The listing builds one solid part. Answer for the finished solid, in the listing's coordinates (mm). A direction names the side the tool comes from. Coordinates: 2 decimals unless noted, no trailing zeros. Order: outer loops, then holes, each group sorted by start corner. A loop starts at its lowest first (then second) coordinate and runs counter-clockwise, first axis right, second up. Notation, with made-up numbers: (34.5, 11) -> (70.5, 11) arc R18 ccw to (70.5, 39) -> close; hole circle Ø1 at (22.25, -36). An arc over 180 degrees is marked (long way). Put each result on its own line as item: value. Start each with the question number.
Autodesk Inventor part; units mm, degrees
ref_plane "YZ Plane" through (0, 0, 0) normal (1, 0, 0) x (0, 1, 0)
ref_plane "XZ Plane" through (0, 0, 0) normal (0, 1, 0) x (-1, 0, 0)
ref_plane "XY Plane" through (0, 0, 0) normal (0, 0, 1) x (1, 0, 0)
sketch "Boceto1" plane through (0, 0, 0) normal (0, 1, 0) x (-1, 0, 0)
  line L0 (20.5, -20.5) -> (-20.5, -20.5)
  line L1 (-20.5, -20.5) -> (-20.5, 20.5)
  line L2 (-20.5, 20.5) -> (20.5, 20.5)
  line L3 (20.5, 20.5) -> (20.5, -20.5)
  point P0 (0, 0)
  point P1 (0, -20.5)
  point P2 (-20.5, 0)
  dimension "d0" = 41
  dimension "d1" = 41
extrude "Extrusión1" add sketch "Boceto1" along normal blind 94
sketch "Boceto2" plane through (0, 94, 0) normal (0, 1, 0) x (1, 0, 0)
  line L0 (20.5, 20.5) -> (-20.5, 20.5)
  line L1 (-20.5, 20.5) -> (59.5, 20.5)
  line L2 (59.5, 20.5) -> (59.5, 6.5)
  line L3 (-20.5, -20.5) -> (20.5, -20.5)
  line L4 (59.5, 6.5) -> (20.5, -20.5)
  line L5 (20.5, -20.5) -> (20.5, 20.5)
  line L6 (50.8333, 0.5) -> (20.5, 0.5)
  line L7 (22.5, 18.5) -> (57.5, 18.5)
  line L8 (57.5, 18.5) -> (57.5, 7.5479)
  line L9 (57.5, 7.5479) -> (50.2086, 2.5)
  line L10 (22.5, 18.5) -> (22.5, 2.5)
  line L11 (22.5, 2.5) -> (50.2086, 2.5)
  line L12 (22.5, 0.5) -> (22.5, -16.6829)
  line L13 (22.5, -16.6829) -> (47.3197, 0.5)
  point P0 (0, 0)
  point P1 (36.3543, 2.5)
  dimension "d4" = 80
  dimension "d5" = 14
  dimension "d9" = 2
  dimension "d10" = 2
  dimension "d11" = 2
  dimension "d12" = 2
  dimension "d13" = 2
  dimension "d20" = 5.0479
extrude "Extrusión2" add sketch "Boceto2" along normal blind 8 contours L1 L2 L4 L6 L5 | L6 L12 L13 L4 L5
sketch "Boceto3" plane through (0, 94, 0) normal (0, 1, 0) x (1, 0, 0)
  line L0 (-20.5, 20.5) -> (-20.5, -20.5)
  line L1 (20.5, -20.5) -> (59.5, 6.5)
  line L2 (-20.5, 20.5) -> (20.5, 20.5)
  line L3 (20.5, 20.5) -> (20.5, -20.5)
  line L4 (20.5, -20.5) -> (-20.5, -20.5)
  line L5 (-20.5, -20.5) -> (-20.5, 20.5)
  point P0 (0, 0)
extrude "Extrusión3" add sketch "Boceto3" along normal blind 8
sketch "Boceto4" plane through (0, 102, 0) normal (0, 1, 0) x (1, 0, 0)
  point P0 (0, 0)
sketch "Boceto6" plane through (0, 102, 0) normal (0, 1, 0) x (1, 0, 0)
  line L0 (-20.5, 20.5) -> (-20.5, -20.5)
  line L1 (59.5, 6.5) -> (59.5, 20.5)
  line L2 (-20.5, 20.5) -> (59.5, 20.5)
  line L3 (59.5, 20.5) -> (59.5, 6.5)
  line L4 (20.5, -20.5) -> (59.5, 6.5)
  line L5 (59.5, 6.5) -> (20.5, -20.5)
  line L6 (20.5, -20.5) -> (-20.5, -20.5)
  line L7 (-20.5, -20.5) -> (-20.5, 20.5)
  point P0 (0, 0)
extrude "Extrusión5" add sketch "Boceto6" along normal blind 1
properties part number "Pata1"
(1) The part is cut by section B-B on x = 33. Determine the outline of the cut face in (y, z).
(2) The part is cut by section C-C on y = 55. Determine the outline of the cut face in (x, z).
(3) A tool of negligible diameter and unlimited length cuts with its end or side. For faces 1 (the flat face through (20.5, 46, 0)), 2 (the flat face through (35, 98, -0.5)), 3 (the flat face through (40, 98, 7)), from which of +Z, -Z, +X, -X, +Y, -Y can it reach the whole face along a straight path? Write none if from no direction.
(4) For a pull along X with two mould halves and no side action, classify faces 4 (the flat face through (10, 103, 0)), 5 (the flat face through (34.74, 97.94, 8.21)), 6 (the flat face through (59.5, 98, -13)), 7 (the flat face through (-20.5, 51, 0)) as released by +X, released by -X, zero draft, split by the parting line, or undercut.
(5) Find the intervals of material crossed by L1, parallel to X at y = 97.5, z = -13.5; L2, parallel to X at y = 88.5, z = 12; L3, parallel to Y at x = 26, z = -8.5, in increasing order.
(6) The part is cut by section A-A on z = -12.5. Determine the outline of the cut face in (x, y).
(7) Each of these flat-tipped pins is pushed along its axis until it touches: P1, Ø8, axis at x = 17.5, z = 7, coming from the -Y side; P2, Ø12.5, axis at y = 33.5, z = -2.5, coming from the +X side; P3, Ø13, axis at x = 44, z = -11, coming from the -Y side; P4, Ø6.5, axis at y = 96.5, z = 4.5, coming from the +X side. Where does it stop, or does it pass through?
(8) The part is cut by section D-D on z = -5. Determine the outline of the cut face in (x, y).
Worked out:
1. outline: (94, -20.5) -> (103, -20.5) -> (103, 11.85) -> (94, 11.85) -> (94, 9.41) -> (102, 9.41) -> (102, -0.5) -> (94, -0.5) -> (94, -2.5) -> (102, -2.5) -> (102, -18.5) -> (94, -18.5) -> close
2. outline: (-20.5, -20.5) -> (20.5, -20.5) -> (20.5, 20.5) -> (-20.5, 20.5) -> close
3. face 1: +Z, -Z, +X, -Y
3. face 2: -Y
3. face 3: +Z, +X, +Y, -Y
4. face 4: zero draft
4. face 5: undercut
4. face 6: released by +X
4. face 7: released by -X
5. L1: -20.5 to 22.5, 57.5 to 59.5
5. L2: -20.5 to 20.5
5. L3: 102 to 103
6. outline: (-20.5, 0) -> (20.5, 0) -> (20.5, 94) -> (22.5, 94) -> (22.5, 102) -> (57.5, 102) -> (57.5, 94) -> (59.5, 94) -> (59.5, 103) -> (-20.5, 103) -> close
7. P1: y = 0
7. P2: x = 20.5
7. P3: y = 102
7. P4: x = 48.31
8. outline: (-20.5, 0) -> (20.5, 0) -> (20.5, 94) -> (22.5, 94) -> (22.5, 102) -> (53.82, 102) -> (53.82, 94) -> (57.33, 94) -> (57.33, 103) -> (-20.5, 103) -> close
